Design review of the part built by this model. Coordinates are the model's own, in mm. Face numbers are marked on the shaded views. A direction names the side the tool comes from. Give positions to 0.01 mm unless a question says otherwise; leave off trailing zeros. Write each loop counter-clockwise with the first axis right and the second up, starting at its lowest first coordinate (ties: lowest second). Pieces come first, ordered by that corner, then holes. Notation, with made-up numbers: (-38, 70.25) -> (-2, 70.25) arc R19 cw to (-2, 103.25) -> close; hole circle Ø11 at (-32, -21.75). An arc over 180 degrees is marked (long way). Use CSV: the item, a comma, the result in double quotes.
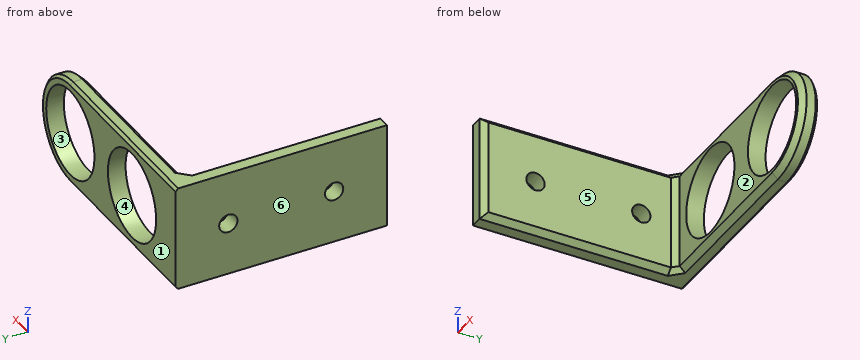
```python
from build123d import *

# Parameters (mm, degrees)
SKETCH1_W           = 38.1
SKETCH1_H           = 38.1
BOSS_EXTRUDE1_DEPTH = 6.35
SKETCH2_R           = 3.302
CUT_EXTRUDE1_DEPTH  = 6.35
SKETCH3_R           = 3.302
CUT_EXTRUDE2_DEPTH  = 6.35
SKETCH4_R           = 15.875
BOSS_EXTRUDE2_DEPTH = 6.35
CHAMFER1_SIZE       = 2.032
CHAMFER2_SIZE       = 1.016


with BuildPart() as part:
    # Sketch1 → Boss-Extrude1 (new body)
    with BuildSketch(Plane(origin=(0, 0, 0), x_dir=(0, 0, -1), z_dir=(1, 0, 0))):
        with Locations((-19.05, 19.05)):
            Rectangle(SKETCH1_W, SKETCH1_H)
        with Locations((-19.05, -19.05)):
            Rectangle(SKETCH1_W, SKETCH1_H)
    extrude(amount=BOSS_EXTRUDE1_DEPTH)

    # Sketch2 → Cut-Extrude1 (cut)
    with BuildSketch(Plane(origin=(6.35, 0, 0), x_dir=(0, 0, -1), z_dir=(1, 0, 0))):
        with Locations((-19.05, -19.05)):
            Circle(SKETCH2_R)
    extrude(amount=-CUT_EXTRUDE1_DEPTH, mode=Mode.SUBTRACT)

    # Sketch3 → Cut-Extrude2 (cut)
    with BuildSketch(Plane(origin=(6.35, 0, 0), x_dir=(0, 0, -1), z_dir=(1, 0, 0))):
        with Locations((-19.05, 19.05)):
            Circle(SKETCH3_R)
    extrude(amount=-CUT_EXTRUDE2_DEPTH, mode=Mode.SUBTRACT)

    # Sketch4 → Boss-Extrude2 (add)
    with BuildSketch(Plane(origin=(0, 38.1, 0), x_dir=(1, 0, 0), z_dir=(0, 1, 0))):
        with BuildLine():
            ThreePointArc((69.215, 0), (88.265, -19.05), (69.215, -38.1))
            Line((69.215, -38.1), (28.575, -38.1))
            Line((28.575, -38.1), (6.35, -38.1))
            Line((6.35, -38.1), (6.35, 0))
            Line((6.35, 0), (28.575, 0))
            Line((28.575, 0), (69.215, 0))
        make_face()
        with Locations((69.215, -19.05)):
            Circle(SKETCH4_R, mode=Mode.SUBTRACT)
        with Locations((28.575, -19.05)):
            Circle(SKETCH4_R, mode=Mode.SUBTRACT)
    extrude(amount=-BOSS_EXTRUDE2_DEPTH)

    # Chamfer1
    chamfer1_edges = [part.edges().sort_by_distance(p)[0] for p in [
        (6.35, -38.1, 19.05),
        (6.35, -3.175, 0),
        (6.35, -3.175, 38.1),
        (37.7825, 31.75, 38.1),
        (88.265, 31.75, 19.05),
        (6.35, 31.75, 19.05),
        (37.7825, 31.75, 0),
    ]]
    chamfer(chamfer1_edges, length=CHAMFER1_SIZE)

    # Chamfer2
    chamfer2_edges = [part.edges().sort_by_distance(p)[0] for p in [
        (34.6075, 38.1, 38.1),
        (88.265, 38.1, 19.05),
        (34.6075, 38.1, 0),
    ]]
    chamfer(chamfer2_edges, length=CHAMFER2_SIZE)


solid = part.part
```
(1) Take a section at A-A (y = 19.05). Write out the cut boundary in (x, z), then the cut area to 3 significant figures.
Established:
outline,"(0, 0) -> (4.32, 0) -> (6.35, 2.03) -> (6.35, 15.75) -> (0, 15.75) -> close; (0, 22.35) -> (6.35, 22.35) -> (6.35, 36.07) -> (4.32, 38.1) -> (0, 38.1) -> close"
area,"196 mm2"
(2) Clearance check with flat-ended pins moving along their axes: pin 1 (5 mm diameter, centred on y = -22.5, z = 22.5, fed in from +X); pin 2 (12 mm diameter, centred on x = 17, y = 4, fed in from -Z); pin 3 (10 mm diameter, centred on x = 53, z = 13, fed in from -Y). State where each tip first meets the part, or that it passes through.
Established:
pin 1,"stops at x = 6.35"
pin 2,"passes through"
pin 3,"stops at y = 31.75"
(3) For line 1 along X through (y, z) = (34, 19); line 2 along Y through (x, z) = (1.5, 19.05); line 3 along Y through (x, z) = (5, 19.05), list the stretches that pass through material, from the lowest coordinate up. Write a range as [from, to].
Established:
line 1,"x = [0, 12.7], [44.45, 53.34], [85.09, 88.26]"
line 2,"y = [-38.1, -22.35], [-15.75, 15.75], [22.35, 38.1]"
line 3,"y = [-37.42, -22.35], [-15.75, 15.75], [22.35, 38.1]"
(4) Mouldability with a two-part tool opening along X and no side actions: class the marked faces 3, 4, 5 and 6 as +X half, -X half, draft (parallel to the pull), parting line (faces both ways), or undercut.
Established:
face 3,"undercut"
face 4,"undercut"
face 5,"+X half"
face 6,"-X half"
(5) Take a section at B-B (z = 19.05). Write out the cut boundary in (x, y) (3 decimals).
Established:
outline,"(0, -38.1) -> (4.318, -38.1) -> (6.35, -36.068) -> (6.35, -22.352) -> (0, -22.352) -> close; (0, -15.748) -> (6.35, -15.748) -> (6.35, 15.748) -> (0, 15.748) -> close; (0, 22.352) -> (6.35, 22.352) -> (6.35, 29.718) -> (8.382, 31.75) -> (12.7, 31.75) -> (12.7, 38.1) -> (0, 38.1) -> close; (44.45, 31.75) -> (53.34, 31.75) -> (53.34, 38.1) -> (44.45, 38.1) -> close; (85.09, 31.75) -> (86.233, 31.75) -> (88.265, 33.782) -> (88.265, 37.084) -> (87.249, 38.1) -> (85.09, 38.1) -> close"
(6) Tool access review of the marked faces 1 and 2: name each direction out of +Z, -Z, +X, -X, +Y, -Y from which nothing blocks a thin tool from reaching the whole face with its end or side.
Established:
face 1,"+Z, -Z, +X, -X, +Y"
face 2,"+Z, -Z, +X, -Y"
(7) Take a section at C-C (x = 49.5). Write out the cut boundary in (y, z).
Established:
outline,"(31.75, 2.03) -> (33.78, 0) -> (37.08, 0) -> (38.1, 1.02) -> (38.1, 37.08) -> (37.08, 38.1) -> (33.78, 38.1) -> (31.75, 36.07) -> close"
(8) Take a section at D-D (x = 23.5). Write out the cut boundary in (y, z).
Established:
outline,"(31.75, 2.03) -> (33.78, 0) -> (37.08, 0) -> (38.1, 1.02) -> (38.1, 4.01) -> (31.75, 4.01) -> close; (31.75, 34.09) -> (38.1, 34.09) -> (38.1, 37.08) -> (37.08, 38.1) -> (33.78, 38.1) -> (31.75, 36.07) -> close"
